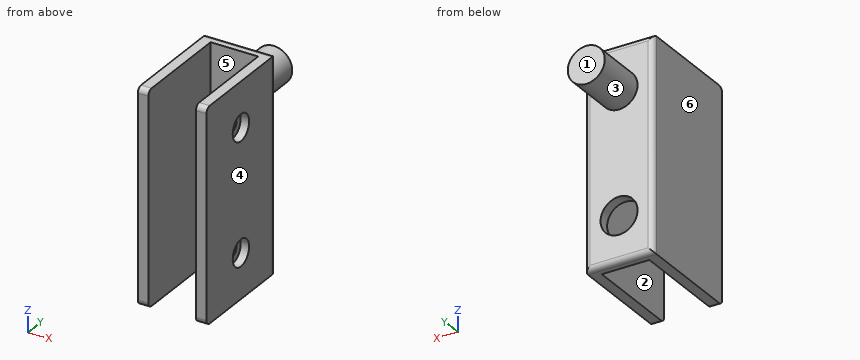
from build123d import *

# Parameters (mm, degrees)
BOSS_EXTRUDE1_DEPTH                              = 20
CBORE_FOR_M2_PAN_HEAD_MACHINE_SCREW1_D           = 2.4
CBORE_FOR_M2_PAN_HEAD_MACHINE_SCREW1_DEPTH       = 2
CBORE_FOR_M2_PAN_HEAD_MACHINE_SCREW1_CBORE_D     = 5
CBORE_FOR_M2_PAN_HEAD_MACHINE_SCREW1_CBORE_DEPTH = 1.6
FILLET1_R                                        = 1
SKETCH4_4_R                                      = 3.5
BOSS_EXTRUDE3_DEPTH                              = 10
SKETCH4_5_R                                      = 3.5
CUT_EXTRUDE2_DEPTH                               = 10


with BuildPart() as part:
    # Sketch1 → Boss-Extrude1 (new, symmetric)
    with BuildSketch(Plane.XY):
        Polygon((-6.5, 21), (-6.5, 0), (-4.5, 0), (-4.5, 19), (0, 19), (0, 21), align=None)
        Polygon((0, 19), (4.5, 19), (4.5, 0), (6.5, 0), (6.5, 21), (0, 21), align=None)
    extrude(amount=BOSS_EXTRUDE1_DEPTH, both=True)

    # CBORE for M2 Pan Head Machine Screw1
    with Locations(Plane(origin=(6.5, 0, 0), x_dir=(0, 0, -1), z_dir=(1, 0, 0))):
        with Locations((-11.5, 10.5), (11.5, 10.5)):
            CounterBoreHole(CBORE_FOR_M2_PAN_HEAD_MACHINE_SCREW1_D / 2, CBORE_FOR_M2_PAN_HEAD_MACHINE_SCREW1_CBORE_D / 2, CBORE_FOR_M2_PAN_HEAD_MACHINE_SCREW1_CBORE_DEPTH, depth=CBORE_FOR_M2_PAN_HEAD_MACHINE_SCREW1_DEPTH)

    # Fillet1
    fillet1_edges = [part.edges().sort_by_distance(p)[0] for p in [
        (-5.5, 0, 20),
        (0, 21, -20),
        (5.5, 0, -20),
        (-5.5, 0, -20),
        (-6.5, 21, 0),
        (6.5, 21, 0),
        (5.5, 0, 20),
        (0, 21, 20),
    ]]
    fillet(fillet1_edges, radius=FILLET1_R)

    # Sketch4<4> → Boss-Extrude3 (add)
    with BuildSketch(Plane(origin=(0, 21, 0), x_dir=(1, 0, 0), z_dir=(0, 1, 0))):
        with Locations(Location((0, -11.5, 0), (0, 0, 90))):
            Circle(SKETCH4_4_R)
    extrude(amount=BOSS_EXTRUDE3_DEPTH)

    # Sketch4<5> → Cut-Extrude2 (cut)
    with BuildSketch(Plane(origin=(0, 21, 0), x_dir=(1, 0, 0), z_dir=(0, 1, 0))):
        with Locations(Location((0, 11.5, 0), (0, 0, 270))):
            Circle(SKETCH4_5_R)
    extrude(amount=-CUT_EXTRUDE2_DEPTH, mode=Mode.SUBTRACT)


solid = part.part
Verification items for the finished model (mm, model axes). Face numbers are marked on the shaded views. A direction names the side the tool comes from. Coordinates: 2 decimals unless noted, no trailing zeros. Loops run counter-clockwise (first coordinate to the right, second up) from the corner with the lowest first, then second, coordinate; pieces in that order, holes last. Notation, with made-up numbers: M 59.5,52.25 L 103.5,52.25 A11 ccw 103.5,64.25 Z; hole C 59,-14 d6. An arc over 180 degrees is marked long. One line per item, written item: value.
1. Section check A-A on z = 11.5. Record the cut outline in (x, y).
Answers follow:
outline: M -6.5,0 L -4.5,0 L -4.5,19 L 4.5,19 L 4.5,11.7 L 4.9,11.7 L 4.9,13 L 6.5,13 L 6.5,20 A1 ccw 5.5,21 L 3.5,21 L 3.5,31 L -3.5,31 L -3.5,21 L -5.5,21 A1 ccw -6.5,20 Z; M 4.5,0 L 6.5,0 L 6.5,8 L 4.9,8 L 4.9,9.3 L 4.5,9.3 Z
2. Section check C-C on y = 6. Record the cut outline in (x, z), plus the area to 3 significant figures.
Answers follow:
outline: M -6.5,-20 L -4.5,-20 L -4.5,20 L -6.5,20 Z; M 4.5,-20 L 6.5,-20 L 6.5,20 L 4.5,20 Z
area: 160 mm^2
3. Section check D-D on z = -11.5. Record the cut outline in (x, y), plus the area to 3 significant figures.
Answers follow:
outline: M -6.5,0 L -4.5,0 L -4.5,19 L -3.5,19 L -3.5,21 L -5.5,21 A1 ccw -6.5,20 Z; M 3.5,19 L 4.5,19 L 4.5,11.7 L 4.9,11.7 L 4.9,13 L 6.5,13 L 6.5,20 A1 ccw 5.5,21 L 3.5,21 Z; M 4.5,0 L 6.5,0 L 6.5,8 L 4.9,8 L 4.9,9.3 L 4.5,9.3 Z
area: 78.6 mm^2
4. Section check B-B on x = 0. Record the cut outline in (y, z).
Answers follow:
outline: M 19,-20 L 20,-20 A1 ccw 21,-19 L 21,-15 L 19,-15 Z; M 19,-8 L 21,-8 L 21,8 L 31,8 L 31,15 L 21,15 L 21,19 A1 ccw 20,20 L 19,20 Z
5. Gauge pin test, flat ends, axial feed: P1, Ø4, axis at y = 9.5, z = -10.5, coming from the +X side; P2, Ø1.5, axis at x = -1, z = 7.5, coming from the -Y side; P3, Ø3, axis at y = 10.5, z = -11.5, coming from the +X side; P4, Ø1.5, axis at x = 3.5, y = 27.5, coming from the -Z side. Record the tip position at first contact, or that the pin passes through.
Answers follow:
P1: x = 6.5
P2: y = 19
P3: x = 4.9
P4: z = 9.33
6. Set-up check for the marked faces 1, 2 and 3: record each of +Z, -Z, +X, -X, +Y, -Y from which the full face is reachable in a straight line by a thin tool's end or side.
Answers follow:
face 1: +Z, -Z, +X, -X, +Y
face 2: +Z, -Z, -Y
face 3: +Y
7. Material ranges on line 1 along X through (y, z) = (11.5, -2); line 2 along Y through (x, z) = (4.8, -11.5); line 3 along Y through (x, z) = (-1, -17), recorded low to high. Write a range as from..to.
Answers follow:
line 1: -6.5..-4.5, 4.5..6.5
line 2: 0..9.3, 11.7..21
line 3: 19..21
8. Mould release check, pull along X, two halves, no side actions. Record for the marked faces 4, 5 and 6: pulls with the +X half, pulls with the -X half, needs draft (parallel to the pull), parting line crosses it, or undercut.
Answers follow:
face 4: pulls with the +X half
face 5: undercut
face 6: pulls with the -X half
